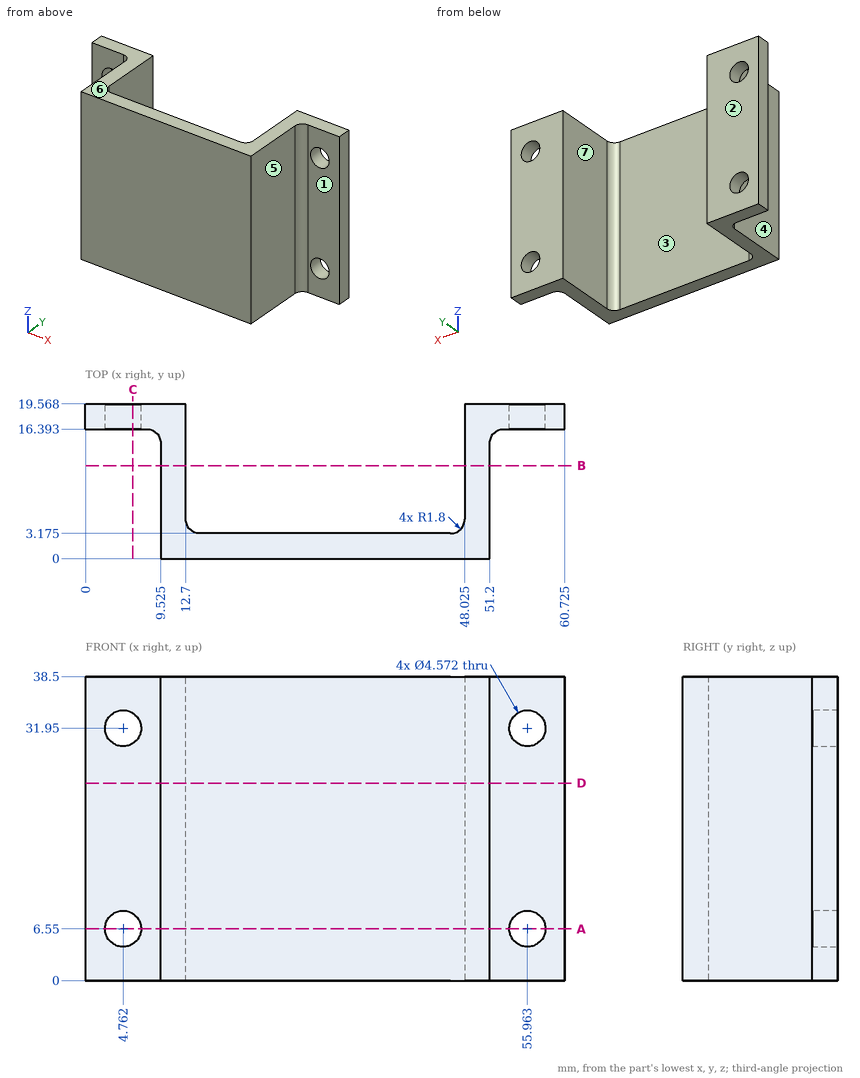
Check sheet for the drawn part. Datum: minimum x, y, z corner. Units: mm. A direction names the side the tool comes from. Coordinates: 2 decimals unless noted, no trailing zeros. Order: outer loops, then holes, each group sorted by start corner. A loop starts at its lowest first (then second) coordinate and runs counter-clockwise, first axis right, second up. Notation, with made-up numbers: M 28.25,51 L 77.25,51 A19 ccw 77.25,56 Z; hole C -10,31 d9. An arc over 180 degrees is marked long. One line per question, with ' | ' between items. Start each with the question number.
Item 1: Gauge pin test, flat ends, axial feed: P1, Ø9.5, axis at x = 37, z = 18.5, coming from the +Y side (1 decimal); P2, Ø4, axis at y = 10.5, z = 20, coming from the -X side (1 decimal); P3, Ø6, axis at x = 58.5, z = 25, coming from the -Y side; P4, Ø4, axis at x = 4.76, z = 31.95, coming from the +Y side. Record the tip position at first contact, or that the pin passes through.
Item 2: Material ranges on line 1 (X direction, y = 17.95, z = 31.95) (1 decimal); line 2 (X direction, y = 7.25, z = 31) (1 decimal); line 3 (Y direction, x = 24, z = 36) (1 decimal), recorded low to high.
Item 3: Sectioned sample at D-D on z = 25. Record the cut outline in (x, y) (1 decimal).
Item 4: Sectioned sample at C-C on x = 6. Record the cut outline in (y, z).
Item 5: Sectioned sample at A-A on z = 6.55. Record the cut outline in (x, y) (1 decimal).
Item 6: Mould release check, pull along X, two halves, no side actions. Record for the marked faces 5, 6 and 7: pulls with the +X half, pulls with the -X half, needs draft (parallel to the pull), parting line crosses it, or undercut.
Item 7: Sectioned sample at B-B on y = 11.75. Record the cut outline in (x, z) (1 decimal).
Item 8: Access from +Z, -Z, +X, -X, +Y, -Y to the whole of each face (thin tool, end or side, straight path). Record for the marked faces 1, 2, 3 and 4.
Answer below:
1) P1: stops at y = 3.2 | P2: stops at x = 9.5 | P3: stops at y = 16.39 | P4: passes through
2) line 1: x = 0 to 2.5, 7 to 12.7, 48 to 53.7, 58.2 to 60.7 | line 2: x = 9.5 to 12.7, 48 to 51.2 | line 3: y = 0 to 3.2
3) outline: M 0,16.4 L 7.7,16.4 A1.8 cw 9.5,14.6 L 9.5,0 L 51.2,0 L 51.2,14.6 A1.8 cw 53,16.4 L 60.7,16.4 L 60.7,19.6 L 48,19.6 L 48,5 A1.8 cw 46.2,3.2 L 14.5,3.2 A1.8 cw 12.7,5 L 12.7,19.6 L 0,19.6 Z
4) outline: M 16.39,0 L 19.57,0 L 19.57,4.63 L 16.39,4.63 Z; M 16.39,8.47 L 19.57,8.47 L 19.57,30.03 L 16.39,30.03 Z; M 16.39,33.87 L 19.57,33.87 L 19.57,38.5 L 16.39,38.5 Z
5) outline: M 0,16.4 L 2.5,16.4 L 2.5,19.6 L 0,19.6 Z; M 7,16.4 L 7.7,16.4 A1.8 cw 9.5,14.6 L 9.5,0 L 51.2,0 L 51.2,14.6 A1.8 cw 53,16.4 L 53.7,16.4 L 53.7,19.6 L 48,19.6 L 48,5 A1.8 cw 46.2,3.2 L 14.5,3.2 A1.8 cw 12.7,5 L 12.7,19.6 L 7,19.6 Z; M 58.2,16.4 L 60.7,16.4 L 60.7,19.6 L 58.2,19.6 Z
6) face 5: pulls with the +X half | face 6: needs draft | face 7: undercut
7) outline: M 9.5,0 L 12.7,0 L 12.7,38.5 L 9.5,38.5 Z; M 48,0 L 51.2,0 L 51.2,38.5 L 48,38.5 Z
8) face 1: +Z, -Z, +X, -Y | face 2: +Z, -Z, +X, -X, +Y | face 3: +Z, -Z, +Y | face 4: +Z, -Z, -X, -Y
